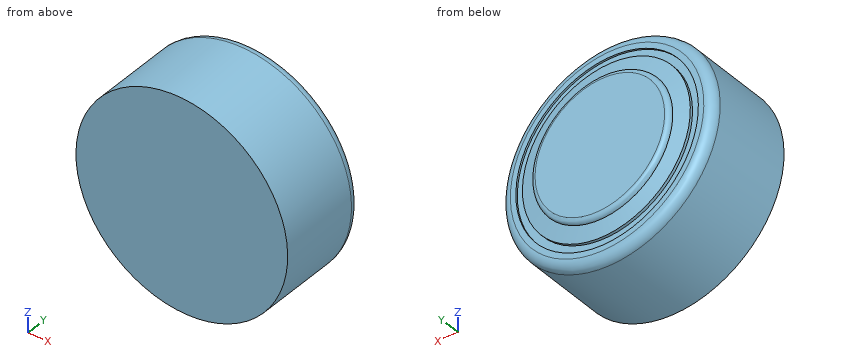
```python
from build123d import *

# Parameters (mm, degrees)
CROQUIS1_R              = 5.8
SALIENTE_EXTRUIR1_DEPTH = 4.9
REDONDEO1_R             = 0.5
CROQUIS2_R              = 5
CORTAR_EXTRUIR1_DEPTH   = 0.1
CROQUIS3_R              = 4.6
SALIENTE_EXTRUIR2_DEPTH = 5.15
CROQUIS4_R              = 3.8
SALIENTE_EXTRUIR3_DEPTH = 5.4
REDONDEO7_R             = 0.25
CHAFL_N1_SIZE           = 0.8
CHAFL_N1_SIZE_2         = 0.2


# Some blends are built 0.0001 mm under size
with BuildPart() as part:
    # Croquis1 → Saliente-Extruir1 (new body)
    with BuildSketch(Plane(origin=(0, 0, 0), x_dir=(1, 0, 0), z_dir=(0, 1, 0))):
        with Locations(Location((0, 0, 0), (0, 0, 270))):
            Circle(CROQUIS1_R)
    extrude(amount=SALIENTE_EXTRUIR1_DEPTH)

    # Redondeo1
    redondeo1_edges = [part.edges().sort_by_distance(p)[0] for p in [
        (0, 4.9, -5.8),
    ]]
    fillet(redondeo1_edges, radius=REDONDEO1_R)

    # Croquis2 → Cortar-Extruir1 (cut)
    with BuildSketch(Plane(origin=(0, 4.9, 0), x_dir=(1, 0, 0), z_dir=(0, 1, 0))):
        with Locations(Location((0, 0, 0), (0, 0, 270))):
            Circle(CROQUIS2_R)
    extrude(amount=-CORTAR_EXTRUIR1_DEPTH, mode=Mode.SUBTRACT)

    # Croquis3 → Saliente-Extruir2 (add)
    with BuildSketch(Plane.XZ):
        with Locations(Location((0, 0, 0), (0, 0, 270))):
            Circle(CROQUIS3_R)
    extrude(amount=-SALIENTE_EXTRUIR2_DEPTH)

    # Croquis4 → Saliente-Extruir3 (add)
    with BuildSketch(Plane.XZ):
        with Locations(Location((0, 0, 0), (0, 0, 270))):
            Circle(CROQUIS4_R)
    extrude(amount=-SALIENTE_EXTRUIR3_DEPTH)

    # Redondeo7
    redondeo7_edges = [part.edges().sort_by_distance(p)[0] for p in [
        (0, 5.4, 3.8),
    ]]
    fillet(redondeo7_edges, radius=REDONDEO7_R - 0.0001)  # a hair under: the kernel refuses the full size

    # Chaflán1
    # the kernel refuses this chamfer: 0.8, 0.2 mm, written as the material it takes off along each edge
    with BuildSketch(Plane(origin=(0, 5.15, 0), x_dir=(0, 0, -1), z_dir=(-1, 0, 0))) as chafl_n1_piece_1_section:
        Polygon((4.6 - CHAFL_N1_SIZE, 0), (4.6, CHAFL_N1_SIZE_2), (4.6, 0), align=None)
    chafl_n1_piece_1 = revolve(axis=Axis((0, 5.15, 0), (0, -1, 0)), mode=Mode.PRIVATE)
    chafl_n1_piece_1 = chafl_n1_piece_1 - Plane(origin=(0, 5.059567154, 0), x_dir=(0, 0, -1), z_dir=(0, -1, 0)) * Cylinder(3.8, 19, mode=Mode.PRIVATE)
    add(chafl_n1_piece_1, mode=Mode.SUBTRACT)


solid = part.part
```
Could you check a few things on this model? Use its own coordinates, in mm. Round coordinates to 2 decimals unless told otherwise and drop trailing zeros. Order: outer loops, then holes, each group sorted by start corner. A loop starts at its lowest first (then second) coordinate and runs counter-clockwise, first axis right, second up. Notation, with made-up numbers: M 84.5,3.25 L 100.5,3.25 A31 cw 100.5,30.25 Z; hole C 55.5,25 d10. An arc over 180 degrees is marked long. One line per question, with ' | ' between items. Start each with the question number.
(1) Suppose I cut it at C-C on y = 3.15. List the corners of the cut face in (x, z) for me, then the cut area to 3 significant figures.
(2) Please list where these lines run through material, in increasing order: line 1 along Y through (x, z) = (2.25, -4.25); line 2 along Y through (x, z) = (-1.5, -5); line 3 along Z through (x, y) = (-1, 2.2).
(3) For P1, Ø1, axis at y = 1.5, z = -1.5, coming from the -X side, with a flat end and sliding along its axis, tell me the tip position at first contact or that it passes through.
Geometry results:
1) outline: C 0,0 d11.6 | area: 106 mm²
2) line 1: 0 to 4.8 | line 2: 0 to 4.9 | line 3: -5.71 to 5.71
3) P1: x = -5.71
